Here's how the part is built. I have some questions about the finished solid (model axes, mm). Face numbers are marked on the shaded views. A direction names the side the tool comes from. Give positions to 0.01 mm unless a question says otherwise; leave off trailing zeros. Write each loop counter-clockwise with the first axis right and the second up, starting at its lowest first coordinate (ties: lowest second). Pieces come first, ordered by that corner, then holes. Notation, with made-up numbers: M 4,9 L 46,9 A17 cw 46,22 Z; hole C 34,-14.75 d9. An arc over 180 degrees is marked long. Use one line per item in the form item = value. Start each with the question number.
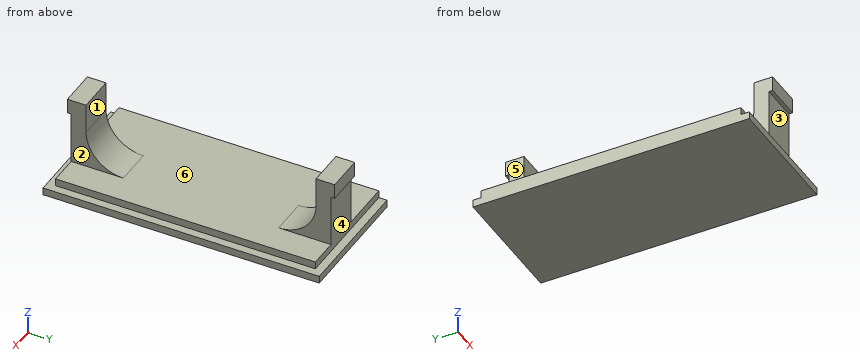
from build123d import *

# Parameters (mm, degrees)
ESQUISSE1_W        = 34
ESQUISSE1_H        = 74
BOSS_EXTRU_1_DEPTH = 2
ESQUISSE2_W        = 31.8
ESQUISSE2_H        = 69.6
BOSS_EXTRU_2_DEPTH = 2
ESQUISSE7_W        = 10
ESQUISSE7_H        = 4
BOSS_EXTRU_5_DEPTH = 18
ESQUISSE8_W        = 10
ESQUISSE8_H        = 1
BOSS_EXTRU_6_DEPTH = 4
CONG_2_R           = 10


with BuildPart() as part:
    # Esquisse1 → Boss.-Extru.1 (new body)
    with BuildSketch(Plane.XY):
        Rectangle(ESQUISSE1_W, ESQUISSE1_H)
    extrude(amount=BOSS_EXTRU_1_DEPTH)

    # Esquisse2 → Boss.-Extru.2 (add)
    with BuildSketch(Plane.XY.offset(2)):
        with Locations((-1.1, 0)):
            Rectangle(ESQUISSE2_W, ESQUISSE2_H)
    extrude(amount=BOSS_EXTRU_2_DEPTH)

    # Esquisse7 → Boss.-Extru.5 (add)
    with BuildSketch(Plane.XY.offset(4)):
        with Locations((2, 32.8)):
            Rectangle(ESQUISSE7_W, ESQUISSE7_H)
        with Locations((2, -32.8)):
            Rectangle(ESQUISSE7_W, ESQUISSE7_H)
    extrude(amount=BOSS_EXTRU_5_DEPTH)

    # Esquisse8 → Boss.-Extru.6 (add)
    with BuildSketch(Plane.XY.offset(22)):
        with Locations((2, 35.3)):
            Rectangle(ESQUISSE8_W, ESQUISSE8_H)
        with Locations((2, -35.3)):
            Rectangle(ESQUISSE8_W, ESQUISSE8_H)
    extrude(amount=-BOSS_EXTRU_6_DEPTH)

    # Congé2
    cong_2_edges = [part.edges().sort_by_distance(p)[0] for p in [
        (2, 30.8, 4),
        (2, -30.8, 4),
    ]]
    fillet(cong_2_edges, radius=CONG_2_R)


solid = part.part
1) Please list where these lines run through material, in increasing order: line 1 (Y direction, x = 6, z = 15.25); line 2 (Z direction, x = 9.5, y = 2.5); line 3 (X direction, y = -16, z = 2.75).
2) On a 3-axis mill with a long thin cutter (end or side, diameter ignored), from which of +Z, -Z, +X, -X, +Y, -Y can I reach the whole of each face in a straight line? I mean the marked faces 1, 2 and 3. Say none if no direction works.
3) Suppose I cut it at A-A, the plane z = 16.75. List the corners of the cut face in (x, y) for me.
4) Will these pins go through, and if not, where does the flat tip stop? P1, Ø2, axis at x = 3.5, z = 19, coming from the +Y side; P2, Ø5, axis at x = -2.5, z = 11.5, coming from the -Y side; P3, Ø7.5, axis at y = -26, z = 9.5, coming from the -X side.
5) Suppose I cut it at B-B, the plane x = 5. List the corners of the cut face in (y, z) for me, and give its area (3 significant figures).
6) Suppose I cut it at C-C, the plane y = -4.5. List the corners of the cut face in (x, z) for me.
7) Suppose I cut it at D-D, the plane z = 20.5. List the corners of the cut face in (x, y) for me, and give its area (3 significant figures).
8) Thinking about a two-plate mould opening in Y: for the marked faces 4, 5 and 6, which applies, released by +Y, released by -Y, zero draft, split by the parting line, or undercut?
Checks:
q1.line_1 = -34.8 to -30.8, 30.8 to 34.8
q1.line_2 = 0 to 4
q1.line_3 = -17 to 14.8
q2.face_1 = +Z, +X, -X
q2.face_2 = +Z, +X, +Y, -Y
q2.face_3 = +X, -X, -Y
q3.outline = M -3,-34.8 L 7,-34.8 L 7,-30.8 L -3,-30.8 Z; M -3,30.8 L 7,30.8 L 7,34.8 L -3,34.8 Z
q4.P1 = 35.8
q4.P2 = -34.8
q4.P3 = -3
q5.outline = M -37,0 L 37,0 L 37,2 L 34.8,2 L 34.8,18 L 35.8,18 L 35.8,22 L 30.8,22 L 30.8,14 A10 cw 20.8,4 L -20.8,4 A10 cw -30.8,14 L -30.8,22 L -35.8,22 L -35.8,18 L -34.8,18 L -34.8,2 L -37,2 Z
q5.area = 482 mm^2
q6.outline = M -17,0 L 17,0 L 17,2 L 14.8,2 L 14.8,4 L -17,4 Z
q7.outline = M -3,-35.8 L 7,-35.8 L 7,-30.8 L -3,-30.8 Z; M -3,30.8 L 7,30.8 L 7,35.8 L -3,35.8 Z
q7.area = 100 mm^2
q8.face_4 = released by +Y
q8.face_5 = zero draft
q8.face_6 = undercut
